CAD build for the part. Positions are in the model's coordinates, mm. A direction names the side the tool comes from. Give positions to 0.01 mm unless a question says otherwise; leave off trailing zeros. Order: outer loops, then holes, each group sorted by start corner. A loop starts at its lowest first (then second) coordinate and runs counter-clockwise, first axis right, second up.
Item 1: Which spindle directions (+Z, -Z, +X, -X, +Y, -Y) get a long thin tool onto all of the face, cutting with end or side? Do faces 4 (the cylindrical face through (-8.486, -0.352, -8.496)), 5 (the flat face through (2, 18, -7.5)), 6 (the flat face through (7, -0.1, -9.4)). Say none if no direction does.
Item 2: Band-saw the part on A-A on y = 0. Give the cut face in (x, z), plus the area to 3 significant figures.
Item 3: Band-saw the part on B-B on x = -3.5. Give the cut face in (y, z).
Item 4: Flat gauge pins, fed straight in: P1, Ø6.5, axis at x = -1, y = -17, coming from the -Z side; P2, Ø6.5, axis at x = 0, y = 16, coming from the -Z side; P3, Ø12, axis at x = 1.5, y = 2.5, coming from the +Z side. Where does each tip first touch, or does it go through?
Item 5: Wall check: L1, parallel to Y at x = 0, z = 2.5; L2, parallel to Y at x = 0, z = -1.75; L3, parallel to Y at x = 7.5, z = 1.5. Give the ranges that are in metal, low to high.
Item 6: Band-saw the part on C-C on z = -3.5. Count the separate pieces of the cut face and the enclosed holes in it, plus the area to 3 significant figures.
Item 7: Two-plate mould, pull along Y, no slides. Class faces 1 (the flat face through (0, -20, 0)), 2 (the cylindrical face through (0, 18, 0)), 3 (the flat face through (2, -18, -7.5)): released by +Y, released by -Y, zero draft, split by the parting line, or undercut.
Item 8: Band-saw the part on D-D on x = -8.5. Give the cut face in (y, z), plus the area to 3 significant figures.
```python
from build123d import *

# Parameters (mm, degrees)
BOSS_EXTRUDE1_DEPTH = 10
BOSS_EXTRUDE2_DEPTH = 7
SKETCH2_R           = 2
CUT_EXTRUDE1_DEPTH  = 15
FILLET1_R           = 0.5


with BuildPart() as part:
    # Sketch1 → Boss-Extrude1 (new, symmetric)
    with BuildSketch(Plane.YZ):
        with BuildLine():
            Line((-10, 7.5), (-16, 7.5))
            ThreePointArc((-16, 7.5), (0, -8.5), (16, 7.5))
            Line((16, 7.5), (10, 7.5))
            ThreePointArc((10, 7.5), (0, -2.5), (-10, 7.5))
        make_face()
    extrude(amount=BOSS_EXTRUDE1_DEPTH, both=True)

    # Sketch1_3 → Boss-Extrude2 (add, symmetric)
    with BuildSketch(Plane.YZ):
        with BuildLine():
            Line((-16, 7.5), (-20, 7.5))
            Line((-20, 7.5), (-20, -7.5))
            Line((-20, -7.5), (-13.228756555, -7.5))
            ThreePointArc((-13.228756555, -7.5), (0, -12.5), (13.228756555, -7.5))
            Line((13.228756555, -7.5), (20, -7.5))
            Line((20, -7.5), (20, 7.5))
            Line((20, 7.5), (16, 7.5))
            ThreePointArc((16, 7.5), (0, -8.5), (-16, 7.5))
        make_face()
    extrude(amount=BOSS_EXTRUDE2_DEPTH, both=True)

    # Sketch2 → Cut-Extrude1 (cut)
    with BuildSketch(Plane.XY.offset(7.5)):
        with Locations((0, 16)):
            Circle(SKETCH2_R)
        with Locations(Location((0, -16, 0), (0, 0, 180))):
            Circle(SKETCH2_R)
    extrude(amount=-CUT_EXTRUDE1_DEPTH, mode=Mode.SUBTRACT)

    # Fillet1
    fillet1_edges = [part.edges().sort_by_distance(p)[0] for p in [
        (10, 0, -8.5),
        (-7, -16.614378278, -7.5),
        (0, -20, -7.5),
        (-7, 0, -12.5),
        (0, -13.228756555, -7.5),
        (-7, 16.614378278, -7.5),
        (0, 13.228756555, -7.5),
        (7, 20, 0),
        (0, 20, -7.5),
        (10, 0, -2.5),
        (7, 0, -8.5),
        (-7, -20, 0),
        (7, -16.614378278, -7.5),
        (7, 0, -12.5),
        (7, 16.614378278, -7.5),
        (7, -20, 0),
        (-7, 0, -8.5),
        (-7, 20, 0),
        (-10, 0, -2.5),
        (-10, 0, -8.5),
    ]]
    fillet(fillet1_edges, radius=FILLET1_R)


solid = part.part
```
The answers:
1. face 4: -Z, -X
1. face 5: -Z, +X, -X, +Y
1. face 6: -Z, +X
2. outline: (-10, -8) arc R0.5 ccw to (-9.5, -8.5) - (-7.5, -8.5) arc R0.5 cw to (-7, -9) - (-7, -12) arc R0.5 ccw to (-6.5, -12.5) - (6.5, -12.5) arc R0.5 ccw to (7, -12) - (7, -9) arc R0.5 cw to (7.5, -8.5) - (9.5, -8.5) arc R0.5 ccw to (10, -8) - (10, -3) arc R0.5 ccw to (9.5, -2.5) - (-9.5, -2.5) arc R0.5 ccw to (-10, -3) - close
2. area: 176 mm2
3. outline: (-20, -7) arc R0.5 ccw to (-19.5, -7.5) - (-13.42, -7.5) arc R0.5 cw to (-13.09, -7.62) arc R20 ccw to (13.09, -7.62) arc R0.5 cw to (13.42, -7.5) - (19.5, -7.5) arc R0.5 ccw to (20, -7) - (20, 7.5) - (10, 7.5) arc R10 cw to (-10, 7.5) - (-20, 7.5) - close
4. P1: stops at z = -7.5
4. P2: stops at z = -7.91
4. P3: stops at z = 2.23
5. L1: y = -20 to -18, -14 to -8.66, 8.66 to 14, 18 to 20
5. L2: y = -20 to -18, -14 to -3.8, 3.8 to 14, 18 to 20
5. L3: y = -14.83 to -8, 8 to 14.83
6. separate pieces: 1
6. enclosed holes: 2
6. area: 674 mm2
7. face 1: released by -Y
7. face 2: undercut
7. face 3: zero draft
8. outline: (-16, 7.5) arc R16 ccw to (16, 7.5) - (10, 7.5) arc R10 cw to (-10, 7.5) - close
8. area: 245 mm2
